The listing builds one solid part. Answer for the finished solid, in the listing's coordinates (mm). A direction names the side the tool comes from. Coordinates: 2 decimals unless noted, no trailing zeros. Loops run counter-clockwise (first coordinate to the right, second up) from the corner with the lowest first, then second, coordinate; pieces in that order, holes last. Notation, with made-up numbers: (2, 19.25) - (22, 19.25) arc R26 cw to (22, 45.25) - close; hole circle Ø5 at (21, 62). An arc over 180 degrees is marked (long way). Return JSON: item names as keys, results as strings. Group by question number.
1. Section D-D (y = 2.75) is taken. Write down the section's boundary in (x, z) (3 decimals), and give its area (3 significant figures).
2. Each of these flat-tipped pins is pushed along its axis until it touches: P1, Ø1.4, axis at x = -11.91, y = 0, coming from the -Z side (3 decimals); P2, Ø4, axis at x = 0, y = -3.97, coming from the +Z side (3 decimals); P3, Ø1.7, axis at x = -12, y = -8, coming from the -Z side. Where does it stop, or does it pass through?
3. Find the intervals of material crossed by line 1 along Y through (x, z) = (0, 3.5); line 2 along X through (y, z) = (0, 8.75) (1 decimal); line 3 along X through (y, z) = (2.25, 5.25) (1 decimal), in increasing order.
4. Which of the six approach directions +Z, -Z, +X, -X, +Y, -Y give full straight-line access (tool end or side, diameter ignored) to faces 5 (the face through (-12, -8, 9.525)), 6 (the face through (5.07, -10.05, 10.31)), 7 (the face through (4, 0, 11.112))?
5. The mould has two halves that part along Y. Classify faces 1 (the face through (9.4, -1.15, 4.02)), 2 (the face through (0, -11.906, 5)), 3 (the face through (12, 0, 11.112)), 4 (the face through (0, 3.969, 5)): pulls with the +Y half, pulls with the -Y half, needs draft (parallel to the pull), parting line crosses it, or undercut.
6. Section A-A (z = 3.5) is taken. State how many separate pieces and enclosed holes the cut face has, and give its area (3 significant figures).
```python
from build123d import *

# Parameters (mm, degrees)
F0_W     = 31.75
F0_H     = 15.875
F0_R     = 2.38125
F1_DEPTH = 9.525
F2_DEPTH = 11.1125
F3_T     = -1.5875
F4_R     = 3.175
F4_R_2   = 2.38125
F5_DEPTH = 7.9375


with BuildPart() as f1:
    # F0 (on Top) → F1 (new body)
    with BuildSketch(Plane.XY):
        with Locations((0, -3.96875)):
            Rectangle(F0_W, F0_H)
        with Locations((-11.90625, -7.9375)):
            Circle(F0_R, mode=Mode.SUBTRACT)
        with Locations((-3.96875, -7.9375)):
            Circle(F0_R, mode=Mode.SUBTRACT)
        with Locations((3.96875, -7.9375)):
            Circle(F0_R, mode=Mode.SUBTRACT)
        with Locations((11.90625, -7.9375)):
            Circle(F0_R, mode=Mode.SUBTRACT)
        with Locations((-11.90625, 0)):
            Circle(F0_R, mode=Mode.SUBTRACT)
        with Locations((-3.96875, 0)):
            Circle(F0_R, mode=Mode.SUBTRACT)
        with Locations((3.96875, 0)):
            Circle(F0_R, mode=Mode.SUBTRACT)
        with Locations((11.90625, 0)):
            Circle(F0_R, mode=Mode.SUBTRACT)
    extrude(amount=F1_DEPTH)

    # F0 (on Top) → F2 (join)
    with BuildSketch(Plane.XY):
        with Locations((-11.90625, 0)):
            Circle(F0_R)
        with Locations((-11.90625, -7.9375)):
            Circle(F0_R)
        with Locations((-3.96875, -7.9375)):
            Circle(F0_R)
        with Locations((-3.96875, 0)):
            Circle(F0_R)
        with Locations((3.96875, 0)):
            Circle(F0_R)
        with Locations((3.96875, -7.9375)):
            Circle(F0_R)
        with Locations((11.90625, -7.9375)):
            Circle(F0_R)
        with Locations((11.90625, 0)):
            Circle(F0_R)
    extrude(amount=F2_DEPTH)

    # F3
    f3_openings = [f1.faces().sort_by_distance(p)[0] for p in [
        (0, -3.96875, 0),
    ]]
    offset(amount=F3_T, openings=f3_openings, kind=Kind.INTERSECTION)

    # F4 (on face) → F5 (join)
    with BuildSketch(Plane(origin=(0, 0, 7.9375), x_dir=(1, 0, 0), z_dir=(0, 0, -1))):
        with BuildLine():
            ThreePointArc((-4.7625, 3.96875), (-6.7224801022, 6.9020675157), (-10.1825640303, 6.2138140303))
            Line((-10.1825640303, 6.2138140303), (-9.6212980227, 5.6525480227))
            ThreePointArc((-9.6212980227, 5.6525480227), (-7.0262350767, 6.1687381368), (-5.55625, 3.96875))
            ThreePointArc((-5.55625, 3.96875), (-5.7375118632, 3.0574850767), (-6.2537019773, 2.2849519773))
            Line((-6.2537019773, 2.2849519773), (-5.6924359697, 1.7236859697))
            ThreePointArc((-5.6924359697, 1.7236859697), (-5.0041824843, 2.7537301022), (-4.7625, 3.96875))
        make_face()
        with BuildLine():
            Line((-9.6212980227, 5.6525480227), (-10.1825640303, 6.2138140303))
            ThreePointArc((-10.1825640303, 6.2138140303), (-10.1825640303, 1.7236859697), (-5.6924359697, 1.7236859697))
            Line((-5.6924359697, 1.7236859697), (-6.2537019773, 2.2849519773))
            ThreePointArc((-6.2537019773, 2.2849519773), (-9.6212980227, 2.2849519773), (-9.6212980227, 5.6525480227))
        make_face()
        with Locations((0, 3.96875)):
            Circle(F4_R)
        with Locations((0, 3.96875)):
            Circle(F4_R_2, mode=Mode.SUBTRACT)
        with Locations((7.9375, 3.96875)):
            Circle(F4_R)
        with Locations((7.9375, 3.96875)):
            Circle(F4_R_2, mode=Mode.SUBTRACT)
    extrude(amount=F5_DEPTH)


solid = f1.part
```
The answers:
{
 "1": {"outline": "(-15.875, 0) - (15.875, 0) - (15.875, 9.525) - (-15.875, 9.525) - close", "area": "302 mm2"},
 "2": {"P1": "stops at z = 9.525", "P2": "stops at z = 9.525", "P3": "stops at z = 7.94"},
 "3": {"line 1": "y = -11.91 to -10.32, -7.14 to -6.35, -1.59 to -0.79, 2.38 to 3.97", "line 2": "x = -15.9 to -12.7, -11.1 to -4.8, -3.2 to 3.2, 4.8 to 11.1, 12.7 to 15.9", "line 3": "x = -15.9 to -14.3, 14.3 to 15.9"},
 "4": {"face 5": "-Z", "face 6": "+Z", "face 7": "+Z, +X, -X, +Y, -Y"},
 "5": {"face 1": "undercut", "face 2": "pulls with the -Y half", "face 3": "needs draft", "face 4": "pulls with the +Y half"},
 "6": {"separate pieces": "4", "enclosed holes": "4", "area": "183 mm2"}
}
